Build history of the part. All positions in model axes, mm. A direction names the side the tool comes from. Round coordinates to 2 decimals unless told otherwise and drop trailing zeros. Write each loop counter-clockwise with the first axis right and the second up, starting at its lowest first coordinate (ties: lowest second). Pieces come first, ordered by that corner, then holes. Notation, with made-up numbers: (61.25, 40.5) -> (118.25, 40.5) arc R13 ccw to (118.25, 45.5) -> close; hole circle Ø5 at (73, 36.5). An arc over 180 degrees is marked (long way). Return JSON: item names as keys, results as strings.
from build123d import *

# Parameters (mm, degrees)
PLATE_EXTRUDE_DEPTH               = 3.81
SKETCH2_R                         = 2.3495
OUTER_HOLE_CUT_DEPTH              = 214.397794272
SKETCH3_R                         = 1.905
ARDUINO_SHAPE_CUT_DEPTH           = 1.905
SKETCH4_W                         = 22.86
SKETCH4_H                         = 29.21
SKETCH4_R                         = 1.905
HG7881_CUT_DEPTH                  = 1.905
SKETCH5_R                         = 1.905
ARDUINO_AND_HG7881_HOLE_CUT_DEPTH = 214.397794272


with BuildPart() as part:
    # Sketch1 → Plate Extrude (new body)
    with BuildSketch(Plane(origin=(0, 0, 0), x_dir=(1, 0, 0), z_dir=(0, 1, 0))):
        with BuildLine():
            Line((6.35, 0), (120.65, 0))
            ThreePointArc((120.65, 0), (125.140128061, 1.859871939), (127, 6.35))
            Line((127, 6.35), (127, 165.1))
            ThreePointArc((127, 165.1), (125.140128061, 169.590128061), (120.65, 171.45))
            Line((120.65, 171.45), (6.35, 171.45))
            ThreePointArc((6.35, 171.45), (1.859871939, 169.590128061), (0, 165.1))
            Line((0, 165.1), (0, 6.35))
            ThreePointArc((0, 6.35), (1.859871939, 1.859871939), (6.35, 0))
        make_face()
    extrude(amount=PLATE_EXTRUDE_DEPTH)

    # Sketch2 → Outer Hole Cut (cut, through all)
    with BuildSketch(Plane(origin=(0, 3.81, 0), x_dir=(1, 0, 0), z_dir=(0, 1, 0))):
        with Locations(Location((6.35, 165.1, 0), (0, 0, 270))):
            Circle(SKETCH2_R)
        with Locations(Location((19.05, 165.1, 0), (0, 0, 270))):
            Circle(SKETCH2_R)
        with Locations(Location((31.75, 165.1, 0), (0, 0, 270))):
            Circle(SKETCH2_R)
        with Locations(Location((44.45, 165.1, 0), (0, 0, 270))):
            Circle(SKETCH2_R)
        with Locations(Location((57.15, 165.1, 0), (0, 0, 270))):
            Circle(SKETCH2_R)
        with Locations(Location((69.85, 165.1, 0), (0, 0, 270))):
            Circle(SKETCH2_R)
        with Locations(Location((82.55, 165.1, 0), (0, 0, 270))):
            Circle(SKETCH2_R)
        with Locations(Location((95.25, 165.1, 0), (0, 0, 270))):
            Circle(SKETCH2_R)
        with Locations(Location((107.95, 165.1, 0), (0, 0, 270))):
            Circle(SKETCH2_R)
        with Locations(Location((120.65, 165.1, 0), (0, 0, 270))):
            Circle(SKETCH2_R)
        with Locations(Location((6.35, 152.4, 0), (0, 0, 270))):
            Circle(SKETCH2_R)
        with Locations(Location((120.65, 152.4, 0), (0, 0, 270))):
            Circle(SKETCH2_R)
        with Locations(Location((6.35, 139.7, 0), (0, 0, 270))):
            Circle(SKETCH2_R)
        with Locations(Location((120.65, 139.7, 0), (0, 0, 270))):
            Circle(SKETCH2_R)
        with Locations(Location((6.35, 127, 0), (0, 0, 270))):
            Circle(SKETCH2_R)
        with Locations(Location((120.65, 127, 0), (0, 0, 270))):
            Circle(SKETCH2_R)
        with Locations(Location((6.35, 114.3, 0), (0, 0, 270))):
            Circle(SKETCH2_R)
        with Locations(Location((120.65, 114.3, 0), (0, 0, 270))):
            Circle(SKETCH2_R)
        with Locations(Location((6.35, 101.6, 0), (0, 0, 270))):
            Circle(SKETCH2_R)
        with Locations(Location((120.65, 101.6, 0), (0, 0, 270))):
            Circle(SKETCH2_R)
        with Locations(Location((6.35, 88.9, 0), (0, 0, 270))):
            Circle(SKETCH2_R)
        with Locations(Location((120.65, 88.9, 0), (0, 0, 270))):
            Circle(SKETCH2_R)
        with Locations(Location((6.35, 76.2, 0), (0, 0, 270))):
            Circle(SKETCH2_R)
        with Locations(Location((120.65, 76.2, 0), (0, 0, 270))):
            Circle(SKETCH2_R)
        with Locations(Location((6.35, 63.5, 0), (0, 0, 270))):
            Circle(SKETCH2_R)
        with Locations(Location((120.65, 63.5, 0), (0, 0, 270))):
            Circle(SKETCH2_R)
        with Locations(Location((6.35, 6.35, 0), (0, 0, 270))):
            Circle(SKETCH2_R)
        with Locations(Location((19.05, 6.35, 0), (0, 0, 270))):
            Circle(SKETCH2_R)
        with Locations(Location((31.75, 6.35, 0), (0, 0, 270))):
            Circle(SKETCH2_R)
        with Locations(Location((44.45, 6.35, 0), (0, 0, 270))):
            Circle(SKETCH2_R)
        with Locations(Location((57.15, 6.35, 0), (0, 0, 270))):
            Circle(SKETCH2_R)
        with Locations(Location((69.85, 6.35, 0), (0, 0, 270))):
            Circle(SKETCH2_R)
        with Locations(Location((82.55, 6.35, 0), (0, 0, 270))):
            Circle(SKETCH2_R)
        with Locations(Location((95.25, 6.35, 0), (0, 0, 270))):
            Circle(SKETCH2_R)
        with Locations(Location((107.95, 6.35, 0), (0, 0, 270))):
            Circle(SKETCH2_R)
        with Locations(Location((120.65, 6.35, 0), (0, 0, 270))):
            Circle(SKETCH2_R)
        with Locations(Location((12.7, 22.225, 0), (0, 0, 270))):
            Circle(SKETCH2_R)
        with Locations(Location((12.7, 34.925, 0), (0, 0, 270))):
            Circle(SKETCH2_R)
        with Locations(Location((12.7, 47.625, 0), (0, 0, 270))):
            Circle(SKETCH2_R)
        with Locations(Location((114.3, 47.625, 0), (0, 0, 270))):
            Circle(SKETCH2_R)
        with Locations(Location((114.3, 34.925, 0), (0, 0, 270))):
            Circle(SKETCH2_R)
        with Locations(Location((114.3, 22.225, 0), (0, 0, 270))):
            Circle(SKETCH2_R)
    extrude(amount=-OUTER_HOLE_CUT_DEPTH, mode=Mode.SUBTRACT)

    # Sketch3 → Arduino Shape Cut (cut)
    with BuildSketch(Plane(origin=(0, 3.81, 0), x_dir=(1, 0, 0), z_dir=(0, 1, 0))):
        Polygon((48.26, 83.566), (81.28, 83.566), (84.074, 86.36), (97.79, 86.36), (97.79, 152.4), (43.18, 152.4), (43.18, 86.36), (45.72, 86.36), align=None)
        with Locations(Location((50.927, 86.106, 0), (0, 0, 270))):
            Circle(SKETCH3_R, mode=Mode.SUBTRACT)
        with Locations(Location((78.867, 86.106, 0), (0, 0, 270))):
            Circle(SKETCH3_R, mode=Mode.SUBTRACT)
        with Locations(Location((45.847, 138.176, 0), (0, 0, 270))):
            Circle(SKETCH3_R, mode=Mode.SUBTRACT)
        with Locations(Location((94.107, 136.906, 0), (0, 0, 270))):
            Circle(SKETCH3_R, mode=Mode.SUBTRACT)
    extrude(amount=-ARDUINO_SHAPE_CUT_DEPTH, mode=Mode.SUBTRACT)

    # Sketch4 → HG7881 Cut (cut)
    # profile 1 of 2: a face of its own
    with BuildSketch(Plane(origin=(0, 3.81, 0), x_dir=(1, 0, 0), z_dir=(0, 1, 0))):
        with Locations((27.94, 141.605)):
            Rectangle(SKETCH4_W, SKETCH4_H)
        with Locations(Location((37.004970647, 137.183397888, 0), (0, 0, 270))):
            Circle(SKETCH4_R, mode=Mode.SUBTRACT)
        with Locations(Location((37.004970647, 150.182885458, 0), (0, 0, 270))):
            Circle(SKETCH4_R, mode=Mode.SUBTRACT)
        with Locations(Location((18.605695933, 150.182885458, 0), (0, 0, 270))):
            Circle(SKETCH4_R, mode=Mode.SUBTRACT)
        with Locations(Location((18.605695933, 137.183397888, 0), (0, 0, 270))):
            Circle(SKETCH4_R, mode=Mode.SUBTRACT)
    # profile 2 of 2: a face of its own
    with BuildSketch(Plane(origin=(0, 3.81, 0), x_dir=(1, 0, 0), z_dir=(0, 1, 0))):
        with Locations((27.94, 97.155)):
            Rectangle(SKETCH4_W, SKETCH4_H)
        with Locations(Location((37.004970647, 92.733397888, 0), (0, 0, 270))):
            Circle(SKETCH4_R, mode=Mode.SUBTRACT)
        with Locations(Location((37.004970647, 105.732885458, 0), (0, 0, 270))):
            Circle(SKETCH4_R, mode=Mode.SUBTRACT)
        with Locations(Location((18.605695933, 105.732885458, 0), (0, 0, 270))):
            Circle(SKETCH4_R, mode=Mode.SUBTRACT)
        with Locations(Location((18.605695933, 92.733397888, 0), (0, 0, 270))):
            Circle(SKETCH4_R, mode=Mode.SUBTRACT)
    extrude(amount=-HG7881_CUT_DEPTH, mode=Mode.SUBTRACT)

    # Sketch5 → Arduino and HG7881 Hole Cut (cut, through all)
    with BuildSketch(Plane(origin=(0, 3.81, 0), x_dir=(1, 0, 0), z_dir=(0, 1, 0))):
        with Locations(Location((94.107, 136.906, 0), (0, 0, 270))):
            Circle(SKETCH5_R)
        with Locations(Location((78.867, 86.106, 0), (0, 0, 270))):
            Circle(SKETCH5_R)
        with Locations(Location((50.927, 86.106, 0), (0, 0, 270))):
            Circle(SKETCH5_R)
        with Locations(Location((45.847, 138.176, 0), (0, 0, 270))):
            Circle(SKETCH5_R)
        with Locations(Location((18.605695933, 150.182885458, 0), (0, 0, 270))):
            Circle(SKETCH5_R)
        with Locations(Location((37.004970647, 150.182885458, 0), (0, 0, 270))):
            Circle(SKETCH5_R)
        with Locations(Location((37.004970647, 137.183397888, 0), (0, 0, 270))):
            Circle(SKETCH5_R)
        with Locations(Location((18.605695933, 137.183397888, 0), (0, 0, 270))):
            Circle(SKETCH5_R)
        with Locations(Location((18.605695933, 105.732885458, 0), (0, 0, 270))):
            Circle(SKETCH5_R)
        with Locations(Location((18.605695933, 92.733397888, 0), (0, 0, 270))):
            Circle(SKETCH5_R)
        with Locations(Location((37.004970647, 92.733397888, 0), (0, 0, 270))):
            Circle(SKETCH5_R)
        with Locations(Location((37.004970647, 105.732885458, 0), (0, 0, 270))):
            Circle(SKETCH5_R)
    extrude(amount=-ARDUINO_AND_HG7881_HOLE_CUT_DEPTH, mode=Mode.SUBTRACT)


solid = part.part
Q1. Pin check, flat tip, straight feed: pin 1 Ø2 at (x, z) = (22, -85.5) entering from +Y (3 decimals). Stop position of the tip, or through.
Verdict:
{"pin 1": "stops at y = 1.905"}
Q2. Saw through at D-D on z = -76.2. List the corners of the cut face in (x, y).
Verdict:
{"outline": "(0, 0) -> (4, 0) -> (4, 3.81) -> (0, 3.81) -> close; (8.7, 0) -> (118.3, 0) -> (118.3, 3.81) -> (8.7, 3.81) -> close; (123, 0) -> (127, 0) -> (127, 3.81) -> (123, 3.81) -> close"}
Q3. Saw through at A-A on x = 69.85. Count the separate pieces of the cut face and the enclosed holes in it, then the cut area to 3 significant figures.
Verdict:
{"separate pieces": "3", "enclosed holes": "0", "area": "486 mm²"}
Q4. Saw through at C-C on x = 114.3. List the corners of the cut face in (y, z), then the cut area to 3 significant figures.
Verdict:
{"outline": "(0, -171.45) -> (3.81, -171.45) -> (3.81, -49.97) -> (0, -49.97) -> close; (0, -45.28) -> (3.81, -45.28) -> (3.81, -37.27) -> (0, -37.27) -> close; (0, -32.58) -> (3.81, -32.58) -> (3.81, -24.57) -> (0, -24.57) -> close; (0, -19.88) -> (3.81, -19.88) -> (3.81, 0) -> (0, 0) -> close", "area": "600 mm²"}
Q5. Two-plate mould, pull along X, no slides. Class faces 3 (the cylindrical face through (5.45, 1.93, -99.43)), 4 (the cylindrical face through (1.81, 1.88, -1.91)), 5 (the cylindrical face through (125.19, 1.88, -169.54)): +X half, -X half, draft (parallel to the pull), parting line (faces both ways), or undercut.
Verdict:
{"face 3": "undercut", "face 4": "-X half", "face 5": "+X half"}
Q6. Saw through at B-B on z = -101.6. List the corners of the cut face in (x, y) (1 decimal), then the cut area to 3 significant figures.
Verdict:
{"outline": "(0, 0) -> (4, 0) -> (4, 3.8) -> (0, 3.8) -> close; (8.7, 0) -> (118.3, 0) -> (118.3, 3.8) -> (97.8, 3.8) -> (97.8, 1.9) -> (43.2, 1.9) -> (43.2, 3.8) -> (39.4, 3.8) -> (39.4, 1.9) -> (16.5, 1.9) -> (16.5, 3.8) -> (8.7, 3.8) -> close; (123, 0) -> (127, 0) -> (127, 3.8) -> (123, 3.8) -> close", "area": "300 mm²"}
Q7. Wall check: L1, parallel to Z at x = 27.5, y = 1.95; L2, parallel to Z at x = 17, y = 1.95; L3, parallel to Z at x = 78, y = 2. Give the ranges that are in metal, low to high.
Verdict:
{"L1": "z = -171.45 to -156.21, -127 to -111.76, -82.55 to 0", "L2": "z = -171.45 to -166.25, -163.95 to -156.21, -127 to -111.76, -82.55 to -7.5, -5.2 to 0", "L3": "z = -171.45 to -152.4, -83.57 to 0"}
Q8. 3-axis set-ups, long thin cutter, end or side, ignore diameter. For faces 1 (the flat face through (70, 1.905, -118)), 2 (the flat face through (64, 2, -171.45)): which of +Z, -Z, +X, -X, +Y, -Y reach the whole face in a straight line?
Verdict:
{"face 1": "+Y", "face 2": "-Z, +X, -X, +Y, -Y"}
